Read the model definition and answer for the solid it produces. Units are mm, in the model's axes. Face numbers are marked on the shaded views. A direction names the side the tool comes from. Give positions to 0.01 mm unless a question says otherwise; leave off trailing zeros. Write each loop counter-clockwise with the first axis right and the second up, starting at its lowest first coordinate (ties: lowest second). Pieces come first, ordered by that corner, then holes. Notation, with made-up numbers: M 24,64 L 77,64 A28 ccw 77,100 Z; hole C -37.75,74.5 d11. An arc over 180 degrees is marked long. Use a Markdown table: item, result. Add a question column.
Item 1: A cutting plane is placed at B-B on y = 51. Determine the outline of the cut face in (x, z).
Item 2: Given P1, Ø0.8, axis at x = 1.5, z = 0.5, coming from the +Y side; P2, Ø0.5, axis at y = 48.5, z = 0.5, coming from the +X side; P3, Ø0.8, axis at x = 13.5, z = 1, coming from the -Y side, each flat-ended and moving along its own axis, determine where each tip first touches the part or whether it passes through.
Item 3: A cutting plane is placed at D-D on x = 4.75. Determine the outline of the cut face in (y, z).
Item 4: The mould has two halves that part along Y. Classify the marked faces 4, 5 and 6: pulls with the +Y half, pulls with the -Y half, needs draft (parallel to the pull), parting line crosses it, or undercut.
Item 5: A cutting plane is placed at C-C on z = 0.85. Count the separate pieces of the cut face and the enclosed holes in it, then the cut area to 3 significant figures.
Item 6: A cutting plane is placed at A-A on x = -6. Determine the outline of the cut face in (y, z), then the cut area to 3 significant figures.
Item 7: Consider probe 1 along X at (y, z) = (49.25, 0.35); probe 2 along Y at (x, z) = (-5.25, 0.55); probe 3 along Y at (x, z) = (7, 1.35). Determine where each line is inside the solid, lowest interval first. Write a range as [from, to].
Item 8: For the marked faces 1, 2 and 3, determine the directions among +Z, -Z, +X, -X, +Y, -Y from which every point of the face is accessible in a straight line to the end or side of a thin tool.
from build123d import *

# Parameters (mm, degrees)
SKETCH1_W           = 1.524
SKETCH1_H           = 1.481764771
SKETCH1_H_2         = 1.524
BOSS_EXTRUDE1_DEPTH = 1.524
SKETCH2_W           = 2.901164826
SKETCH2_H           = 1.524
CUT_EXTRUDE1_DEPTH  = 1.524


with BuildPart() as part:
    # Sketch1 → Boss-Extrude1 (new body)
    with BuildSketch(Plane.XY):
        with BuildLine():
            Line((-9.201867242, 66.283387572), (-4.791154517, 62.964734812))
            Line((-4.791154517, 62.964734812), (-3.874879328, 64.182526165))
            Line((-3.874879328, 64.182526165), (-7.967249174, 67.261655396))
            ThreePointArc((-7.967249174, 67.261655396), (-9.053535436, 69.319058784), (-9.439830642, 71.613334825))
            ThreePointArc((-9.439830642, 71.613334825), (-7.929515653, 69.608329431), (-5.454408435, 69.190068442))
            ThreePointArc((-5.454408435, 69.190068442), (-1.979913279, 68.569755109), (1.547610416, 68.453643912))
            ThreePointArc((1.547610416, 68.453643912), (2.250493371, 67.501534847), (3.14522315, 66.726928661))
            ThreePointArc((3.14522315, 66.726928661), (7.095824067, 66.377438321), (10.638674299, 64.594854987))
            ThreePointArc((10.638674299, 64.594854987), (13.932057854, 60.788978675), (14.582785292, 55.798224871))
            ThreePointArc((14.582785292, 55.798224871), (12.199808945, 50.134207473), (7.917480129, 45.72724375))
            ThreePointArc((7.917480129, 45.72724375), (3.14522315, 43.837178873), (-1.890077483, 44.833436601))
            ThreePointArc((-1.890077483, 44.833436601), (-6.113668677, 48.360365036), (-8.490380039, 53.323145493))
            ThreePointArc((-8.490380039, 53.323145493), (-8.760469415, 54.639184362), (-9.439830642, 55.798224871))
            ThreePointArc((-9.439830642, 55.798224871), (-9.784898441, 59.308308116), (-9.439830642, 62.818391362))
            ThreePointArc((-9.439830642, 62.818391362), (-10.203506988, 64.594854987), (-11.563650446, 65.969276447))
            ThreePointArc((-11.563650446, 65.969276447), (-10.417196882, 66.385269605), (-9.201867242, 66.283387572))
        make_face()
        Polygon((-1.502614608, 64.205247413), (0, 64.205247413), (0, 62.684788315), (-1.519736188, 62.684788315), align=None, mode=Mode.SUBTRACT)
        with Locations((-0.762, 51.153972349)):
            Rectangle(SKETCH1_W, SKETCH1_H, mode=Mode.SUBTRACT)
        with Locations((6.945775543, 61.8002372)):
            Rectangle(SKETCH1_W, SKETCH1_H_2, mode=Mode.SUBTRACT)
        with Locations((1.55818596, 48.853678484)):
            Rectangle(SKETCH1_W, SKETCH1_H_2, mode=Mode.SUBTRACT)
    extrude(amount=BOSS_EXTRUDE1_DEPTH)

    # Sketch2 → Cut-Extrude1 (cut)
    with BuildSketch(Plane.XY.offset(1.524)):
        Polygon((10.838910474, 47.694983966), (9.113748292, 49.563912383), (7.993907093, 48.530214319), (9.719069274, 46.661285901), align=None)
        with Locations((13.841078696, 55.662305548)):
            Rectangle(SKETCH2_W, SKETCH2_H)
    extrude(amount=-CUT_EXTRUDE1_DEPTH, mode=Mode.SUBTRACT)


solid = part.part
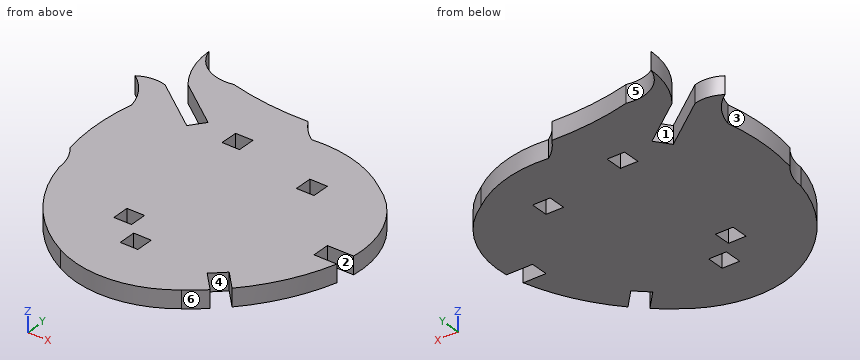
Filled in:
| question | item | result |
|---|---|---|
| 1 | outline | M -7.7,0 L -1.52,0 L -1.52,1.52 L -7.7,1.52 Z; M 0,0 L 12.74,0 L 12.74,1.52 L 0,1.52 Z |
| 2 | P1 | y = 68.45 |
| 2 | P2 | x = 11.18 |
| 2 | P3 | y = 51.67 |
| 3 | outline | M 44.13,0 L 66.77,0 L 66.77,1.52 L 44.13,1.52 Z |
| 4 | face 4 | undercut |
| 4 | face 5 | pulls with the +Y half |
| 4 | face 6 | pulls with the -Y half |
| 5 | separate pieces | 1 |
| 5 | enclosed holes | 4 |
| 5 | area | 456 mm² |
| 6 | outline | M 48.22,0 L 63.87,0 L 63.87,1.52 L 48.22,1.52 Z; M 65.78,0 L 69.12,0 L 69.12,1.52 L 65.78,1.52 Z |
| 6 | area | 28.9 mm² |
| 7 | probe 1 | [-6.75, 0.8], [2.32, 8.77], [9.4, 11.57] |
| 7 | probe 2 | [47.36, 63.31], [65.22, 69.14] |
| 7 | probe 3 | [45.1, 61.04], [62.56, 66.4] |
| 8 | face 1 | +Z, -Z |
| 8 | face 2 | +Z, -Z, +X |
| 8 | face 3 | +Z, -Z, -X |
